Here's how the part is built. I have some questions about the finished solid (model axes, mm). Face numbers are marked on the shaded views. A direction names the side the tool comes from. Give positions to 0.01 mm unless a question says otherwise; leave off trailing zeros. Loops run counter-clockwise (first coordinate to the right, second up) from the corner with the lowest first, then second, coordinate; pieces in that order, holes last. Notation, with made-up numbers: M 50.5,-24 L 85.5,-24 A16 cw 85.5,-16 Z; hole C -26.5,41.25 d1. An arc over 180 degrees is marked long. Answer as CSV lines item,"result". Start each with the question number.
Item 1: If we mould it in two halves opening along X, with no side actions, what happens to the marked faces 1, 2, 3 and 4? For each: released by +X, released by -X, zero draft, split by the parting line, or undercut.
Item 2: I want a section at A-A on y = -5. List the corners of the cut face in (x, z) for me (1 decimal), plus the area to 3 significant figures.
Item 3: If I drill on line 1 along Y through (x, z) = (0, 3.5); line 2 along Y through (x, z) = (-6, 2); line 3 along X through (y, z) = (7, 3.75), over which ranges is the centre line in solid material (lowest first)? Write a range as from..to.
Item 4: I want a section at D-D on y = -14. List the corners of the cut face in (x, z) for me (1 decimal).
Item 5: I want a section at C-C on y = 2.5. List the corners of the cut face in (x, z) for me (3 decimals).
Item 6: Will these pins go through, and if not, where does the flat tip stop? P1, Ø3, axis at x = -14.29, z = 4.76, coming from the -Y side; P2, Ø2, axis at x = -10, z = 5, coming from the +Y side; P3, Ø3.5, axis at x = 14.29, z = 4.76, coming from the +Y side.
Item 7: For the marked faces 5 and 6, which set-ups out of +Z, -Z, +X, -X, +Y, -Y let a thin tool reach every point of the face, with its end or its side?
Item 8: I want a section at B-B on x = 0. List the corners of the cut face in (y, z) for me (1 decimal).
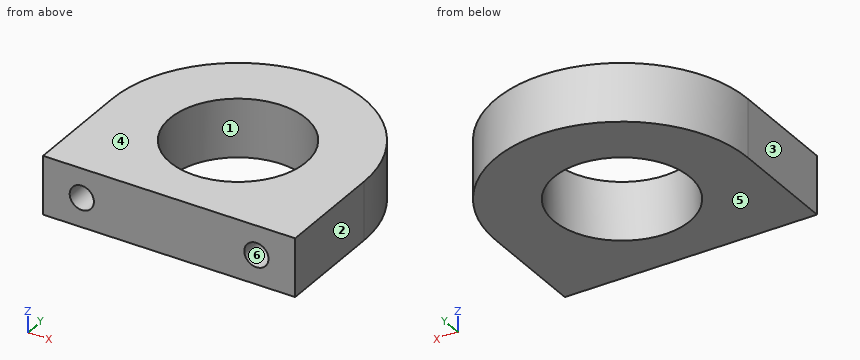
Autodesk Inventor part; units mm, degrees
ref_plane "YZ Plane" through (0, 0, 0) normal (1, 0, 0) x (0, 1, 0)
ref_plane "XZ Plane" through (0, 0, 0) normal (0, 1, 0) x (-1, 0, 0)
ref_plane "XY Plane" through (0, 0, 0) normal (0, 0, 1) x (1, 0, 0)
sketch "Sketch1" plane through (0, 0, 0) normal (0, 0, 1) x (1, 0, 0)
  circle A0 centre (0, 0) radius 11.1125
  arc A1 (20.6375, 0) -> (-20.6375, 0) centre (0, 0) ccw
  line L0 (20.6375, 0) -> (20.6375, -17.907)
  line L1 (20.6375, -17.907) -> (-20.6375, -17.907)
  line L2 (-20.6375, -17.907) -> (-20.6375, 0)
  dimension "d0" = 22.225
  dimension "d2" = 9.525
  dimension "d3" = 17.907
extrude "Extrusion1" add sketch "Sketch1" along normal blind 9.525
sketch "Sketch2" plane through (-20.6375, -17.907, 0) normal (0, -1, 0) x (1, 0, 0)
  circle A0 centre (6.35, 4.7625) radius 2.8195
  circle A1 centre (34.925, 4.7625) radius 2.8195
  line L0 (0, 0) -> (0, 9.525)
  line L1 (41.275, 0) -> (41.275, 9.525)
  point P0 (20.6375, 0)
  point P1 (0, 4.7625)
  point P2 (41.275, 4.7625)
  dimension "d6" = 5.639
  dimension "d7" = 6.35
  dimension "d8" = 6.35
hole "Hole1" at (-14.2875, -17.907, 4.7625) at (14.2875, -17.907, 4.7625) direction (0, 1, 0) diameter 3.9624 depth 13.6144 tip angle 118
properties part number "3DPRINT,VERTICAL,ROLLER,TOP,BEARING,BLOCK"
Result:
1,face 1,"undercut"
1,face 2,"released by +X"
1,face 3,"released by -X"
1,face 4,"zero draft"
2,outline,"M -20.6,0 L -9.9,0 L -9.9,9.5 L -20.6,9.5 Z; M 9.9,0 L 20.6,0 L 20.6,9.5 L 9.9,9.5 Z; hole C -14.3,4.8 d4; hole C 14.3,4.8 d4"
2,area,"179 mm^2"
3,line 1,"-17.91..-11.11, 11.11..20.64"
3,line 2,"-17.91..-9.35, 9.35..19.75"
3,line 3,"-19.41..-8.63, 8.63..19.41"
4,outline,"M -20.6,0 L 20.6,0 L 20.6,9.5 L -20.6,9.5 Z; hole C -14.3,4.8 d4; hole C 14.3,4.8 d4"
5,outline,"M -20.486,0 L -10.828,0 L -10.828,9.525 L -20.486,9.525 Z; M 10.828,0 L 20.486,0 L 20.486,9.525 L 10.828,9.525 Z"
6,P1,"y = -4.01"
6,P2,"y = 18.57"
6,P3,"y = 16.39"
7,face 5,"-Z, +X, -X, +Y, -Y"
7,face 6,"-Y"
8,outline,"M -17.9,0 L -11.1,0 L -11.1,9.5 L -17.9,9.5 Z; M 11.1,0 L 20.6,0 L 20.6,9.5 L 11.1,9.5 Z"
